For this review, take the finished solid that the model builds, in its own axes (mm). Coordinates: 2 decimals unless noted, no trailing zeros. Loops run counter-clockwise (first coordinate to the right, second up) from the corner with the lowest first, then second, coordinate; pieces in that order, holes last. Notation, with made-up numbers: (-19, 79.25) - (6, 79.25) arc R18 cw to (6, 104.25) - close; hole circle Ø11 at (85.25, -20). An arc over 180 degrees is marked (long way). Answer as a JSON object with one key per item and string values. Group by question number.
Item 1: We need section A-A (x = -71). Give the boundary of the cut face in (y, z).
Item 2: To check wall thickness, follow line 1 (Z direction, x = 45.5, y = -55). State the ranges of the line that lie inside material, in increasing order.
Item 3: Clearance check with flat-ended pins moving along their axes: pin 1 (8 mm diameter, centred on y = -114.5, z = 36.5, fed in from -X); pin 2 (1.5 mm diameter, centred on x = 81, z = 47.5, fed in from +Y); pin 3 (6 mm diameter, centred on x = -21, y = -61, fed in from -Z). State where each tip first meets the part, or that it passes through.
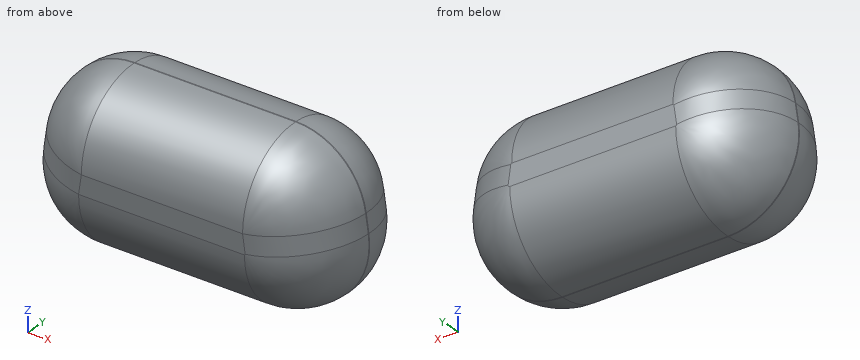
from build123d import *

# Parameters (mm, degrees)
PAD001_DEPTH = 150
FILLET002_R  = 75
FILLET003_R  = 74


with BuildPart() as part:
    # Sketch009 → Pad001 (new body)
    with BuildSketch(Plane.XZ):
        with BuildLine():
            Line((-85.222763, 170), (85.222763, 170))
            ThreePointArc((159.424699, 105.912049), (134.246208, 151.760037), (85.222763, 170))
            Line((162.229991, 86.83606), (159.424699, 105.912049))
            ThreePointArc((87.229991, 0), (144.6005, 26.255941), (162.229991, 86.83606))
            Line((87.229991, 0), (-88.16394, 0))
            ThreePointArc((-162.365875, 85.912049), (-144.923977, 25.976555), (-88.16394, 0))
            Line((-159.424699, 105.912049), (-162.365875, 85.912049))
            ThreePointArc((-85.222763, 170), (-134.246208, 151.760037), (-159.424699, 105.912049))
        make_face()
    extrude(amount=PAD001_DEPTH)

    # Fillet002
    fillet002_edges = [part.edges().sort_by_distance(p)[0] for p in [
        (-134.246208, -150, 151.760037),
        (0, -150, 170),
        (134.246208, -150, 151.760037),
        (160.827345, -150, 96.374055),
        (144.6005, -150, 26.255941),
        (-0.466974, -150, 0),
        (-144.923977, -150, 25.976555),
        (-160.895287, -150, 95.912049),
    ]]
    fillet(fillet002_edges, radius=FILLET002_R)

    # Fillet003
    fillet003_edges = [part.edges().sort_by_distance(p)[0] for p in [
        (-134.246208, 0, 151.760037),
        (0, 0, 170),
        (134.246208, 0, 151.760037),
        (160.827345, 0, 96.374055),
        (144.6005, 0, 26.255941),
        (-0.466974, 0, 0),
        (-144.923977, 0, 25.976555),
        (-160.895287, 0, 95.912049),
    ]]
    fillet(fillet003_edges, radius=FILLET003_R)


solid = part.part
Check sheet entries:
{
 "1": {"outline": "(-150, 75) arc R75 ccw to (-75, 0) - (-74, 0) arc R74 ccw to (0, 74) - (0, 96) arc R74 ccw to (-74, 170) - (-75, 170) arc R75 ccw to (-150, 95) - close"},
 "2": {"line 1": "z = 2.48 to 167.52"},
 "3": {"pin 1": "stops at x = -143.01", "pin 2": "stops at y = -4.62", "pin 3": "stops at z = 0.68"}
}
